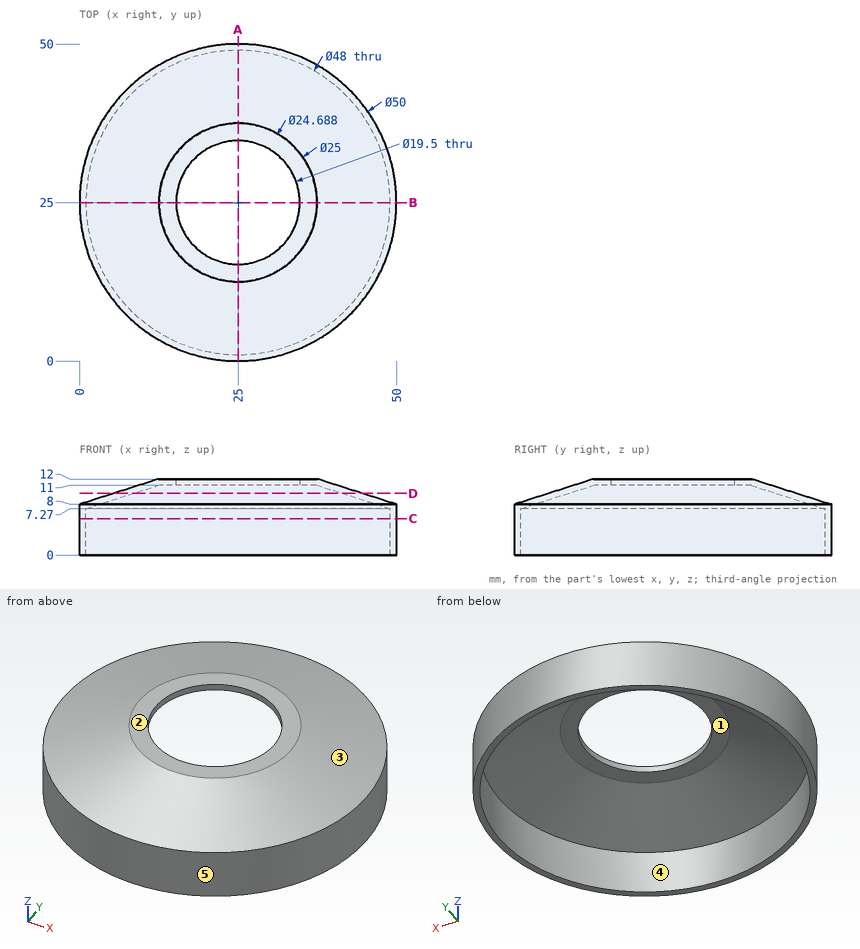
Job drawing, mm, ordinate dimensions from the low corner. One solid piece. A direction names the side the tool comes from. Round coordinates to 2 decimals unless told otherwise and drop trailing zeros. Loops run counter-clockwise (first coordinate to the right, second up) from the corner with the lowest first, then second, coordinate; pieces in that order, holes last. Notation, with made-up numbers: (-11.75, -24.5) -> (34.25, -24.5) arc R10 ccw to (34.25, -20.5) -> close; hole circle Ø2 at (26, -37). An arc over 180 degrees is marked (long way). Use CSV: the item, a comma, the result in double quotes. Start each with the question number.
Q1. Saw through at D-D on z = 9.75. Give the cut face in (x, y).
Q2. Flat gauge pins, fed straight in: pin 1 Ø5 at (y, z) = (32.5, 2.5) entering from -X (3 decimals); pin 2 Ø1.5 at (x, y) = (42, 11.5) entering from +Z; pin 3 Ø20 at (x, y) = (30, 21) entering from -Z. Where does each tip first touch, or does it go through?
Q3. Mould opens along Y. For the marked faces 1, 2 and 3 say: +Y half, -Y half, draft (parallel to the pull), parting line (faces both ways), or undercut.
Q4. Which spindle directions (+Z, -Z, +X, -X, +Y, -Y) get a long thin tool onto all of the face, cutting with end or side? Do the marked faces 4 and 5. Say none if no direction does.
Q5. Saw through at C-C on z = 5.75. Give the cut face in (x, y).
Q6. Saw through at A-A on x = 25. Give the cut face in (y, z).
Q7. Drill centre lines: L1, parallel to Y at x = 25, z = 5.5; L2, parallel to Y at x = 33, z = 0.75 (1 decimal); L3, parallel to X at y = 5.5, z = 3 (1 decimal). Where is each one in solid material? Low to high.
Solutions:
1,outline,"circle Ø39.06 at (25, 25); hole circle Ø32.5 at (25, 25)"
2,pin 1,"stops at x = 0.505"
2,pin 2,"stops at z = 9.29"
2,pin 3,"stops at z = 9.7"
3,face 1,"undercut"
3,face 2,"draft"
3,face 3,"parting line"
4,face 4,"-Z"
4,face 5,"+Z, -Z"
5,outline,"circle Ø50 at (25, 25); hole circle Ø48 at (25, 25)"
6,outline,"(0, 0) -> (1, 0) -> (1, 7.27) -> (12.66, 11) -> (15.25, 11) -> (15.25, 12) -> (12.5, 12) -> (0, 8) -> close; (34.75, 11) -> (37.34, 11) -> (49, 7.27) -> (49, 0) -> (50, 0) -> (50, 8) -> (37.5, 12) -> (34.75, 12) -> close"
7,L1,"y = 0 to 1, 49 to 50"
7,L2,"y = 1.3 to 2.4, 47.6 to 48.7"
7,L3,"x = 9.4 to 11, 39 to 40.6"
